The model under review builds one solid part; all positions refer to its coordinate system, in mm. A direction names the side the tool comes from. Coordinates: 2 decimals unless noted, no trailing zeros. Write each loop counter-clockwise with the first axis right and the second up, starting at its lowest first coordinate (ties: lowest second). Pieces come first, ordered by that corner, then holes.
```python
from build123d import *

# Parameters (mm, degrees)
F0_W        = 76.3128548861
F0_H        = 76.6920521855
F1_DEPTH    = 25.4
F2_T1_DEPTH = 189.756750182
F3_T1_DEPTH = 143.7659818188
F4_R        = 8.9325225018
F6_D        = 12.7
F7_W        = 16.36798447
F7_H        = 35.9481759369
F8_DEPTH    = 17.526


# Not quite as in the source:
# - a fillet or chamfer that OpenCascade refuses, or shapes differently, is made with other operations: its cross-section is extruded or revolved along the edge and cut away or added


with BuildPart() as f1:
    # F0 (on Front) → F1 (new body)
    with BuildSketch(Plane.XZ):
        with Locations((38.156427443, -38.3460260928)):
            Rectangle(F0_W, F0_H)
    extrude(amount=F1_DEPTH)

    # F2: fillet of radius 22.6887790592 on 2 edges, made by hand

    # F2_s2 → F2_t1 (cut)
    with BuildSketch(Plane.YZ.offset(-56.721947648)):
        with BuildLine():
            ThreePointArc((-2.7112209408, 0), (-18.7546104704, -6.6453895296), (-25.4, -22.6887790592))
            Line((-25.4, -22.6887790592), (-25.4, 0))
            Line((-25.4, 0), (-2.7112209408, 0))
        make_face()
        with BuildLine():
            ThreePointArc((-22.6887790592, 0), (-6.6453895296, -6.6453895296), (0, -22.6887790592))
            Line((0, -22.6887790592), (0, 0))
            Line((0, 0), (-22.6887790592, 0))
        make_face()
    extrude(amount=F2_T1_DEPTH, mode=Mode.SUBTRACT)

    # F3: fillet of radius 13.4906253865 on 2 edges, made by hand

    # F3_s2 → F3_t1 (cut)
    with BuildSketch(Plane.YZ.offset(-33.7265634664)):
        with BuildLine():
            ThreePointArc((-25.4, -63.201426799), (-21.4486873067, -72.7407394923), (-11.9093746135, -76.6920521855))
            Line((-11.9093746135, -76.6920521855), (-25.4, -76.6920521855))
            Line((-25.4, -76.6920521855), (-25.4, -63.201426799))
        make_face()
        with BuildLine():
            ThreePointArc((0, -63.201426799), (-3.9513126933, -72.7407394923), (-13.4906253865, -76.6920521855))
            Line((-13.4906253865, -76.6920521855), (0, -76.6920521855))
            Line((0, -76.6920521855), (0, -63.201426799))
        make_face()
    extrude(amount=F3_T1_DEPTH, mode=Mode.SUBTRACT)

    # F4
    f4_edges = [f1.edges().sort_by_distance(p)[0] for p in [
        (38.156427, -12.7, -2.317108),
    ]]
    fillet(f4_edges, radius=F4_R)

    # F6 (through all)
    with Locations(Plane.YZ.offset(76.3128548861)):
        with Locations((-12.2666405514, -16.3046810776)):
            Hole(F6_D / 2)

    # F7 (on face) → F8 (join)
    with BuildSketch(Plane.YZ.offset(76.3128548861)):
        with Locations((-12.4732137192, -44.8362212628)):
            Rectangle(F7_W, F7_H)
    extrude(amount=F8_DEPTH)


solid = f1.part
```
Item 1: Take a section at C-C, the plane x = 80. Write out the cut boundary in (y, z), plus the area to 3 significant figures.
Solved:
outline: (-20.66, -62.81) - (-4.29, -62.81) - (-4.29, -26.86) - (-20.66, -26.86) - close
area: 588 mm2
Item 2: To check wall thickness, follow line 1 along X through (y, z) = (-21, -30.5); line 2 along Z through (x, y) = (8.5, -9); line 3 along Z through (x, y) = (31.5, -7.25). State the ranges of each line that lie inside material, in increasing order.
Solved:
line 1: x = 0 to 76.31
line 2: z = -75.92 to -21.75, -10.86 to -5.1
line 3: z = -75.16 to -20.2, -12.41 to -6.15
Item 3: Take a section at A-A, the plane z = -19.5. Write out the cut boundary in (x, y).
Solved:
outline: (0, -25.17) - (76.31, -25.17) - (76.31, -17.75) - (0, -17.75) - close; (0, -6.78) - (76.31, -6.78) - (76.31, -0.23) - (0, -0.23) - close
Item 4: For pin 1 (3 mm diameter, centred on x = 71.5, y = -20, fed in from -Z); pin 2 (13 mm diameter, centred on x = 86.5, y = -11, fed in from -Z); pin 3 (5 mm diameter, centred on x = 10, y = -3.5, fed in from -Z), all flat-tipped, find the tip position at first contact; note any pin that passes through.
Solved:
pin 1: stops at z = -74.97
pin 2: stops at z = -62.81
pin 3: stops at z = -74.42
Item 5: Mouldability with a two-part tool opening along Y and no side actions: class faces 1 (the face through (37.622, -23.745, -14.181)), 2 (the face through (37.622, -18.323, -14.397)), 3 (the face through (0, -13, -41)), 4 (the face through (37.622, -3.578, -72.353)) as pulls with the +Y half, pulls with the -Y half, needs draft (parallel to the pull), parting line crosses it, or undercut.
Solved:
face 1: pulls with the -Y half
face 2: undercut
face 3: needs draft
face 4: pulls with the +Y half
Item 6: Take a section at B-B, the plane z = -54.5. Write out the cut boundary in (x, y), plus the area to 3 significant figures.
Solved:
outline: (0, -25.4) - (76.31, -25.4) - (76.31, -20.66) - (93.84, -20.66) - (93.84, -4.29) - (76.31, -4.29) - (76.31, 0) - (0, 0) - close
area: 2,230 mm2
Item 7: Take a section at D-D, the plane y = -23. Write out the cut boundary in (x, z), plus the area to 3 significant figures.
Solved:
outline: (0, -70.88) - (76.31, -70.88) - (76.31, -12.53) - (0, -12.53) - close
area: 4,450 mm2
Item 8: Machinability: for faces 5 (the face through (85, -20.657, -45)), 6 (the face through (85, -4.289, -45)), 7 (the face through (85, -13, -62.81)), which of the approach directions +Z, -Z, +X, -X, +Y, -Y give a long, thin tool a straight path to every point of the face, cutting with its end or side? Answer none if there is none.
Solved:
face 5: +Z, -Z, +X, -Y
face 6: +Z, -Z, +X, +Y
face 7: -Z, +X, +Y, -Y
